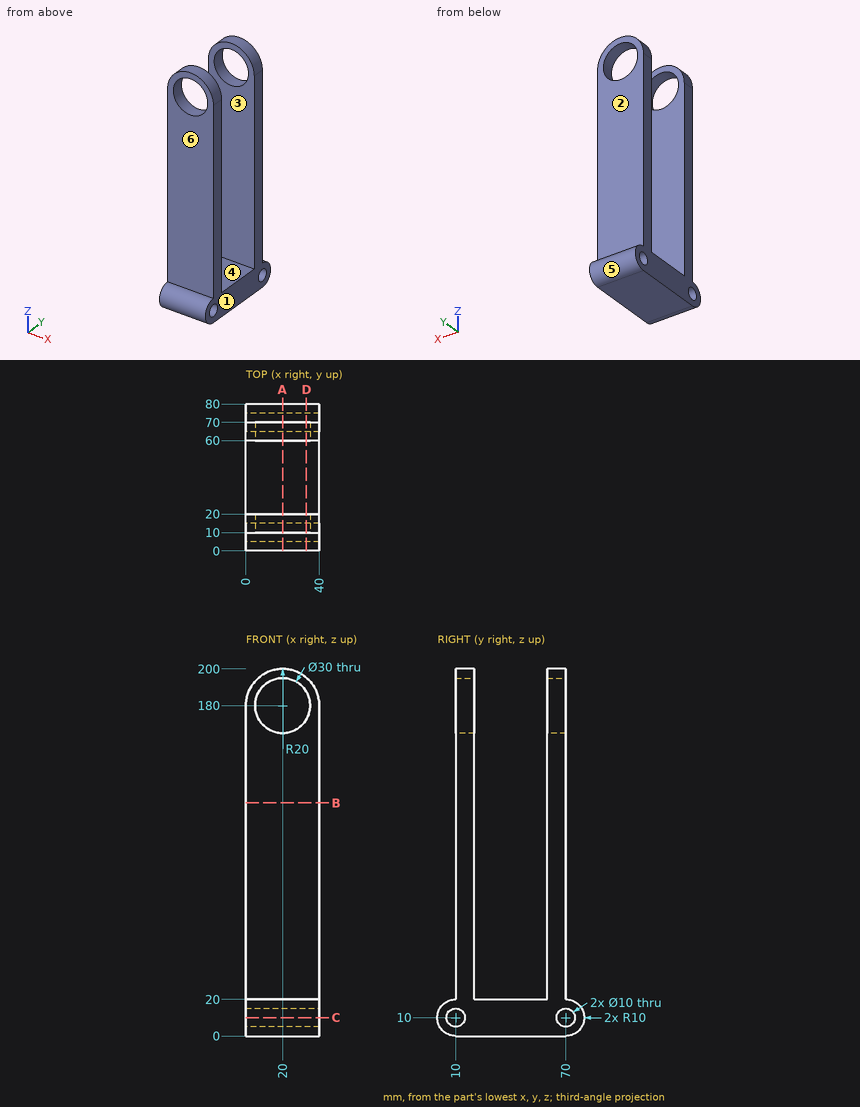
Job drawing, mm, ordinate dimensions from the low corner. One solid piece. A direction names the side the tool comes from. Coordinates: 2 decimals unless noted, no trailing zeros. Write each loop counter-clockwise with the first axis right and the second up, starting at its lowest first coordinate (ties: lowest second). Pieces come first, ordered by that corner, then holes. Notation, with made-up numbers: (46, 76.5) - (104, 76.5) arc R18 ccw to (104, 102.5) - close; hole circle Ø1 at (9, -6.75). An arc over 180 degrees is marked (long way). Use a Markdown table: item, result. Add a question column.
Item 1: Flat gauge pins, fed straight in: pin 1 (12 mm diameter, centred on x = 29, z = 142.5, fed in from -Y); pin 2 (4 mm diameter, centred on x = 8, y = 16.5, fed in from +Z); pin 3 (20 mm diameter, centred on x = 28, z = 149, fed in from +Y). Where does each tip first touch, or does it go through?
Item 2: Band-saw the part on D-D, the plane x = 33. Give the cut face in (y, z), and give its area (3 significant figures).
Item 3: Drill centre lines: L1, parallel to Y at x = 22, z = 10; L2, parallel to X at y = 67.5, z = 180; L3, parallel to Y at x = 28, z = 61. Where is each one in solid material? Low to high. Write a range as from..to.
Item 4: 3-axis set-ups, long thin cutter, end or side, ignore diameter. For the marked faces 1, 2 and 3: which of +Z, -Z, +X, -X, +Y, -Y reach the whole face in a straight line?
Item 5: Band-saw the part on B-B, the plane z = 127. Give the cut face in (x, y).
Item 6: Band-saw the part on A-A, the plane x = 20. Give the cut face in (y, z), and give its area (3 significant figures).
Item 7: Mould opens along Y. For the marked faces 4, 5 and 6 say: pulls with the +Y half, pulls with the -Y half, needs draft (parallel to the pull), parting line crosses it, or undercut.
Item 8: Band-saw the part on C-C, the plane z = 10. Give the cut face in (x, y).
Numbers:
| question | item | result |
|---|---|---|
| 1 | pin 1 | y = 10 |
| 1 | pin 2 | z = 197.32 |
| 1 | pin 3 | y = 70 |
| 2 | outline | (10, 0) - (70, 0) arc R10 ccw to (70, 20) - (70, 172.52) - (60, 172.52) - (60, 20) - (20, 20) - (20, 172.52) - (10, 172.52) - (10, 20) arc R10 ccw to start; (10, 187.48) - (20, 187.48) - (20, 195.2) - (10, 195.2) - close; (60, 187.48) - (70, 187.48) - (70, 195.2) - (60, 195.2) - close; hole circle Ø10 at (10, 10); hole circle Ø10 at (70, 10) |
| 2 | area | 4,560 mm2 |
| 3 | L1 | 0..5, 15..65, 75..80 |
| 3 | L2 | 0..5, 35..40 |
| 3 | L3 | 10..20, 60..70 |
| 4 | face 1 | +Z, -Z, +X, +Y, -Y |
| 4 | face 2 | +Z, +X, -X, +Y |
| 4 | face 3 | +Z, +X, -X |
| 5 | outline | (0, 10) - (40, 10) - (40, 20) - (0, 20) - close; (0, 60) - (40, 60) - (40, 70) - (0, 70) - close |
| 6 | outline | (10, 0) - (70, 0) arc R10 ccw to (70, 20) - (70, 165) - (60, 165) - (60, 20) - (20, 20) - (20, 165) - (10, 165) - (10, 20) arc R10 ccw to start; (10, 195) - (20, 195) - (20, 200) - (10, 200) - close; (60, 195) - (70, 195) - (70, 200) - (60, 200) - close; hole circle Ø10 at (10, 10); hole circle Ø10 at (70, 10) |
| 6 | area | 4,360 mm2 |
| 7 | face 4 | undercut |
| 7 | face 5 | pulls with the +Y half |
| 7 | face 6 | pulls with the -Y half |
| 8 | outline | (0, 0) - (40, 0) - (40, 5) - (0, 5) - close; (0, 15) - (40, 15) - (40, 65) - (0, 65) - close; (0, 75) - (40, 75) - (40, 80) - (0, 80) - close |
